Geometry: final body of the model. Coordinates: model frame, mm. Face numbers are marked on the shaded views. A direction names the side the tool comes from. Coordinates: 2 decimals unless noted, no trailing zeros. Order: outer loops, then holes, each group sorted by start corner. A loop starts at its lowest first (then second) coordinate and runs counter-clockwise, first axis right, second up. Notation, with made-up numbers: M 13,-16 L 43,-16 A23 cw 43,17 Z; hole C 4.5,6 d3. An arc over 180 degrees is marked long. Use CSV: the item, a comma, the result in double quotes. Start each with the question number.
1. Set-up query: the marked faces 4, 5 and 6. Return all of +Z, -Z, +X, -X, +Y, -Y with unobstructed straight access to the full face (end or side cutting, diameter ignored); none if empty.
2. Section query B-B on y = -35.5. Return the cut outline in (x, z).
3. Pull-direction query (Z, two-part tool) for the marked faces 1, 2 and 3; classes: pulls with the +Z half, pulls with the -Z half, needs draft (parallel to the pull), parting line crosses it, or undercut.
4. Section query A-A on y = -2.5. Return the cut outline in (x, z).
5. First-contact query: P1, Ø6, axis at x = 0.5, z = -2, coming from the +Y side; P2, Ø1.5, axis at x = -8, y = -2, coming from the +Z side; P3, Ø0.6, axis at x = -13.5, z = 2, coming from the +Y side; P4, Ø13.5, axis at x = 0, z = 0, coming from the +Y side. Flat tips, straight axial feed; report the tip coordinate or a pass-through.
6. Section query D-D on y = -18. Return the cut outline in (x, z), and give its area (3 significant figures).
7. Material intervals for line 1 (Z direction, x = 0, y = 1); line 2 (Y direction, x = -9.5, z = -3.25), sorted ascending.
8. Section query C-C on y = -29. Return the cut outline in (x, z).
from build123d import *

# Parameters (mm, degrees)
SKETCH1_R                        = 14
BOSS_EXTRUDE1_DEPTH              = 6
SKETCH2_R                        = 14
BOSS_EXTRUDE2_DEPTH              = 15
SKETCH3_R                        = 10
BOSS_EXTRUDE3_DEPTH              = 31
F_10_5_10_5_DIAMETER_HOLE1_D     = 10.5
F_10_5_10_5_DIAMETER_HOLE1_DEPTH = 22
F_10_5_10_5_DIAMETER_HOLE1_TIP   = 3.15451825
CHAMFER1_SIZE                    = 1
SKETCH5_W                        = 6.241360462
SKETCH5_H                        = 33.57083513
SKETCH5_W_2                      = 3.803761641
CUT_EXTRUDE2_DEPTH               = 10
SKETCH6_W                        = 1.2
SKETCH6_H                        = 2


with BuildPart() as part:
    # Sketch1 → Boss-Extrude1 (new body)
    with BuildSketch(Plane(origin=(0, 0, 0), x_dir=(1, 0, 0), z_dir=(0, 1, 0))):
        Circle(SKETCH1_R)
    extrude(amount=BOSS_EXTRUDE1_DEPTH)

    # Sketch2 → Boss-Extrude2 (add)
    with BuildSketch(Plane.XZ):
        Circle(SKETCH2_R)
    extrude(amount=BOSS_EXTRUDE2_DEPTH)

    # Sketch3 → Boss-Extrude3 (add)
    with BuildSketch(Plane.XZ.offset(15)):
        Circle(SKETCH3_R)
    extrude(amount=BOSS_EXTRUDE3_DEPTH)

    # Ø10.5 (10.5) Diameter Hole1
    with Locations(Plane.ZX.offset(6)):
        with Locations((0, 0)):
            Hole(F_10_5_10_5_DIAMETER_HOLE1_D / 2, depth=F_10_5_10_5_DIAMETER_HOLE1_DEPTH)
            with Locations((0, 0, -(F_10_5_10_5_DIAMETER_HOLE1_DEPTH + F_10_5_10_5_DIAMETER_HOLE1_TIP / 2))):  # 118° drill point
                Cone(0, F_10_5_10_5_DIAMETER_HOLE1_D / 2, F_10_5_10_5_DIAMETER_HOLE1_TIP, mode=Mode.SUBTRACT)

    # Chamfer1
    chamfer1_edges = [part.edges().sort_by_distance(p)[0] for p in [
        (-10, -46, 0),
    ]]
    chamfer(chamfer1_edges, length=CHAMFER1_SIZE)

    # Sketch5 → Cut-Extrude2 (cut)
    with BuildSketch(Plane(origin=(0, 6, 0), x_dir=(1, 0, 0), z_dir=(0, 1, 0))):
        with Locations((-15.020680231, 0)):
            Rectangle(SKETCH5_W, SKETCH5_H)
        with Locations((13.801880821, 0)):
            Rectangle(SKETCH5_W_2, SKETCH5_H)
    extrude(amount=-CUT_EXTRUDE2_DEPTH, mode=Mode.SUBTRACT)

    # Sketch6 → Cut-Revolve1 (revolve, cut)
    with BuildSketch(Plane(origin=(0, 0, 0), x_dir=(0, 0, -1), z_dir=(1, 0, 0))):
        with Locations((-10, -35.6)):
            Rectangle(SKETCH6_W, SKETCH6_H)
    revolve(axis=Axis((0, -46, 0), (0, 1, 0)), mode=Mode.SUBTRACT)


solid = part.part
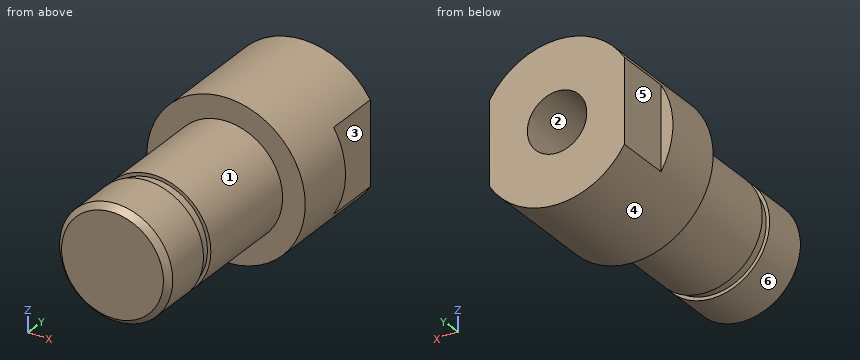
Results list:
1,face 4,"+Y, -Y"
1,face 5,"+Z, -Z, -X, +Y"
1,face 6,"-Y"
2,outline,"C 0,0 d18.8"
3,face 1,"parting line crosses it"
3,face 2,"undercut"
3,face 3,"needs draft"
4,outline,"M -11.9,-7.37 A14 ccw 11.9,-7.37 L 11.9,7.37 A14 ccw -11.9,7.37 Z; hole C 0,0 d10.5"
5,P1,"stops at y = -16.11"
5,P2,"stops at z = 11.98"
5,P3,"stops at y = -4"
5,P4,"stops at y = 6"
6,outline,"C 0,0 d20; hole C 0,0 d3.84"
6,area,"303 mm²"
7,line 1,"z = -14 to -5.25, 5.25 to 14"
7,line 2,"y = -15 to 6"
8,outline,"C 0,0 d20"
